```python
from build123d import *

# Parameters (mm, degrees)
REVOLVE1_ANGLE          = 180
CUT_EXTRUDE1_REACH      = 71.236
CUT_EXTRUDE1_END_RADIUS = 18.04
SKETCH2_R               = 2.8


with BuildPart() as part:
    # Sketch1 → Revolve1 (revolve)
    with BuildSketch(Plane.XY):
        Polygon((40.76425, 22.1), (36.125, 22.1), (36.125, 12.3), (46.125, 12.3), (46.125, 22.1), align=None)
    revolve(axis=Axis((53.3, 30.34, 0), (-1, 0, 0)), revolution_arc=REVOLVE1_ANGLE)

    # Cut-Extrude1: up to this cylinder (the profile starts inside it)
    cut_extrude1_end = Plane(origin=(41.125, 30.34, 0), z_dir=(1, 0, 0)) * Cylinder(CUT_EXTRUDE1_END_RADIUS, 179.552, mode=Mode.PRIVATE)
    # Sketch2 → Cut-Extrude1 (cut, up to the surface)
    with BuildSketch(Plane(origin=(0, 0, 0), x_dir=(-1, 0, 0), z_dir=(0, 0, -1)), mode=Mode.PRIVATE) as cut_extrude1_sk1:
        with Locations((-41.125, 43.48)):
            Circle(SKETCH2_R)
    cut_extrude1_tool1 = extrude(cut_extrude1_sk1.sketch, amount=-CUT_EXTRUDE1_REACH, mode=Mode.PRIVATE) & cut_extrude1_end
    add(cut_extrude1_tool1.solids().sort_by_distance((41.125, 43.48, 0))[0], mode=Mode.SUBTRACT)
    # Sketch2 → Cut-Extrude1 (cut, up to the surface)
    with BuildSketch(Plane(origin=(0, 0, 0), x_dir=(-1, 0, 0), z_dir=(0, 0, -1)), mode=Mode.PRIVATE) as cut_extrude1_sk2:
        with Locations((-41.125, 17.281263544)):
            Circle(SKETCH2_R)
    cut_extrude1_tool2 = extrude(cut_extrude1_sk2.sketch, amount=-CUT_EXTRUDE1_REACH, mode=Mode.PRIVATE) & cut_extrude1_end
    add(cut_extrude1_tool2.solids().sort_by_distance((41.125, 17.281264, 0))[0], mode=Mode.SUBTRACT)


solid = part.part
```
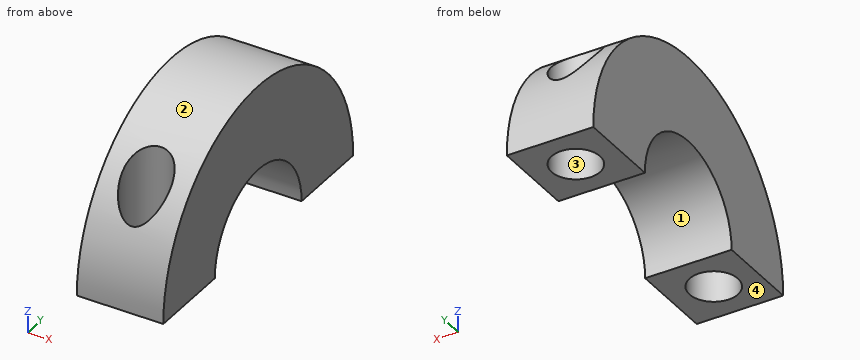
Geometry: final body of the model. Coordinates: model frame, mm. Face numbers are marked on the shaded views. Coordinates: 2 decimals unless noted, no trailing zeros. Order: outer loops, then holes, each group sorted by start corner. A loop starts at its lowest first (then second) coordinate and runs counter-clockwise, first axis right, second up. Notation, with made-up numbers: M 49,75.25 L 75,75.25 A21 cw 75,80.25 Z; hole C -13.5,13 d6. An arc over 180 degrees is marked long. Answer in a Markdown table with one row per item. Add a question column.
Q1. Section query C-C on y = 45.5. Return the cut outline in (x, z) (3 decimals).
Q2. Section query A-A on z = 2.25. Return the cut outline in (x, y) (3 decimals).
Q3. Line query: L1, parallel to Y at x = 39.5, z = 5.5; L2, parallel to Y at x = 39, z = 2; L3, parallel to X at y = 43.48, z = 3.5 (3 decimals). Output: solid intervals per line, ascending.
Q4. Mould query, pull axis Y, two halves, no side actions, for the marked faces 1, 2, 3 and 4. Classes: released by +Y, released by -Y, zero draft, split by the parting line, or undercut.
Q5. Contact query for flat-ended pins moving along their axis: P1, Ø1, axis at x = 43.5, y = 26.5, coming from the -Z side; P2, Ø6, axis at y = 27.5, z = 6, coming from the +X side (3 decimals); P3, Ø4, axis at x = 42.5, z = 3, coming from the -Y side. Output: stop coordinate, or through.
Q6. Section query B-B on x = 42. Return the cut outline in (y, z).
Q7. Section query D-D on z = 9.25. Return the cut outline in (x, y) (3 decimals).
Completed:
| question | item | result |
|---|---|---|
| 1 | outline | M 36.125,0 L 39.186,0 L 39.186,9.778 L 36.125,9.778 Z; M 43.064,0 L 46.125,0 L 46.125,9.778 L 43.064,9.778 Z |
| 2 | outline | M 36.125,12.441 L 46.125,12.441 L 46.125,22.413 L 36.125,22.413 Z; M 36.125,38.267 L 46.125,38.267 L 46.125,48.239 L 36.125,48.239 Z; hole C 41.125,17.281 d5.6; hole C 41.125,43.48 d5.6 |
| 3 | L1 | y = 13.16 to 15, 19.56 to 24.2, 36.48 to 41.2, 45.76 to 47.52 |
| 3 | L2 | y = 12.41 to 15.46, 19.1 to 22.35, 38.33 to 41.66, 45.3 to 48.27 |
| 3 | L3 | x = 36.125 to 38.325, 43.925 to 46.125 |
| 4 | face 1 | undercut |
| 4 | face 2 | split by the parting line |
| 4 | face 3 | undercut |
| 4 | face 4 | zero draft |
| 5 | P1 | stops at z = 7 |
| 5 | P2 | stops at x = 46.125 |
| 5 | P3 | stops at y = 12.33 |
| 6 | outline | M 12.3,0 L 14.62,0 L 14.62,8.85 A18.04 ccw Z; M 19.94,0 L 22.1,0 A8.24 cw 38.58,0 L 40.82,0 L 40.82,14.68 A18.04 ccw 19.94,14.74 Z; M 46.14,0 L 48.38,0 A18.04 ccw 46.14,8.71 Z |
| 7 | outline | M 36.125,14.852 L 39.733,14.852 A2.8 cw long 42.517,14.852 L 46.125,14.852 L 46.125,45.828 L 42.65,45.828 A2.8 cw long 39.6,45.828 L 36.125,45.828 Z |
